Build history of the part. All positions in model axes, mm. Give positions to 0.01 mm unless a question says otherwise; leave off trailing zeros. Order: outer loops, then holes, each group sorted by start corner. A loop starts at its lowest first (then second) coordinate and runs counter-clockwise, first axis right, second up. Notation, with made-up numbers: (-20, -11) - (-2, -11) arc R3 ccw to (-2, -7) - close; hole circle Ø11 at (26.5, -34). An arc over 180 degrees is marked (long way). Use a Markdown table: item, result.
from build123d import *

# Parameters (mm, degrees)
SKETCH1_R           = 60
SKETCH1_R_2         = 31
SKETCH1_R_3         = 3.25
BOSS_EXTRUDE1_DEPTH = 1.5


with BuildPart() as part:
    # Sketch1 → Boss-Extrude1 (new body)
    with BuildSketch(Plane.XY):
        Circle(SKETCH1_R)
        Circle(SKETCH1_R_2, mode=Mode.SUBTRACT)
        with Locations((0, 51.6)):
            Circle(SKETCH1_R_3, mode=Mode.SUBTRACT)
        with Locations((30.329719018, 41.74527691)):
            Circle(SKETCH1_R_3, mode=Mode.SUBTRACT)
        with Locations((49.074516241, 15.94527691)):
            Circle(SKETCH1_R_3, mode=Mode.SUBTRACT)
        with Locations((49.074516241, -15.94527691)):
            Circle(SKETCH1_R_3, mode=Mode.SUBTRACT)
        with Locations((30.329719018, -41.74527691)):
            Circle(SKETCH1_R_3, mode=Mode.SUBTRACT)
        with Locations((0, -51.6)):
            Circle(SKETCH1_R_3, mode=Mode.SUBTRACT)
        with Locations((-30.329719018, -41.74527691)):
            Circle(SKETCH1_R_3, mode=Mode.SUBTRACT)
        with Locations((-49.074516241, -15.94527691)):
            Circle(SKETCH1_R_3, mode=Mode.SUBTRACT)
        with Locations((-49.074516241, 15.94527691)):
            Circle(SKETCH1_R_3, mode=Mode.SUBTRACT)
        with Locations((-30.329719018, 41.74527691)):
            Circle(SKETCH1_R_3, mode=Mode.SUBTRACT)
    extrude(amount=BOSS_EXTRUDE1_DEPTH)


solid = part.part
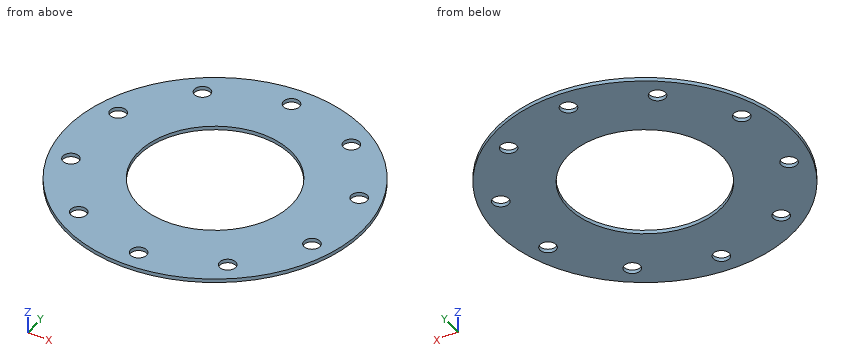
1) Slice it at A-A (y = 0). Write the cut outline in (x, z), and give its area (3 significant figures).
Computed:
| item | result |
|---|---|
| outline | (-60, 0) - (-31, 0) - (-31, 1.5) - (-60, 1.5) - close; (31, 0) - (60, 0) - (60, 1.5) - (31, 1.5) - close |
| area | 87.0 mm² |
2) Slice it at D-D (x = 23.5). Write the cut outline in (y, z), and give its area (3 significant figures).
Computed:
| item | result |
|---|---|
| outline | (-55.21, 0) - (-20.22, 0) - (-20.22, 1.5) - (-55.21, 1.5) - close; (20.22, 0) - (55.21, 0) - (55.21, 1.5) - (20.22, 1.5) - close |
| area | 105 mm² |
3) Slice it at C-C (z = 1.05). State how many separate pieces and enclosed holes the cut face has, and give its area (3 significant figures).
Computed:
| item | result |
|---|---|
| separate pieces | 1 |
| enclosed holes | 11 |
| area | 7,960 mm² |
4) Pin check, flat tips, straight feed: P1, Ø10.5, axis at x = 0, y = -51.6, coming from the -Z side; P2, Ø4, axis at x = 30.33, y = -41.75, coming from the +Z side. Stop position of each tip, or through.
Computed:
| item | result |
|---|---|
| P1 | stops at z = 0 |
| P2 | passes through |
5) Wall check: line 1 (Y direction, x = -3, z = 0.15); line 2 (X direction, y = -14.5, z = 1.2); line 3 (Y direction, x = 49, z = 1.1). Give the ranges that are in metal, low to high. Write a range as from..to.
Computed:
| item | result |
|---|---|
| line 1 | y = -59.92..-52.85, -50.35..-30.85, 30.85..50.35, 52.85..59.92 |
| line 2 | x = -58.22..-51.99, -46.16..-27.4, 27.4..46.16, 51.99..58.22 |
| line 3 | y = -34.63..-19.19, -12.7..12.7, 19.19..34.63 |
6) Slice it at B-B (x = 0). Write the cut outline in (y, z).
Computed:
| item | result |
|---|---|
| outline | (-60, 0) - (-54.85, 0) - (-54.85, 1.5) - (-60, 1.5) - close; (-48.35, 0) - (-31, 0) - (-31, 1.5) - (-48.35, 1.5) - close; (31, 0) - (48.35, 0) - (48.35, 1.5) - (31, 1.5) - close; (54.85, 0) - (60, 0) - (60, 1.5) - (54.85, 1.5) - close |
